Could you check a few things on this drawing? It's one solid part, dimensions in mm from its lowest x, y, z. Coordinates: 2 decimals unless noted, no trailing zeros. Order: outer loops, then holes, each group sorted by start corner. A loop starts at its lowest first (then second) coordinate and runs counter-clockwise, first axis right, second up.
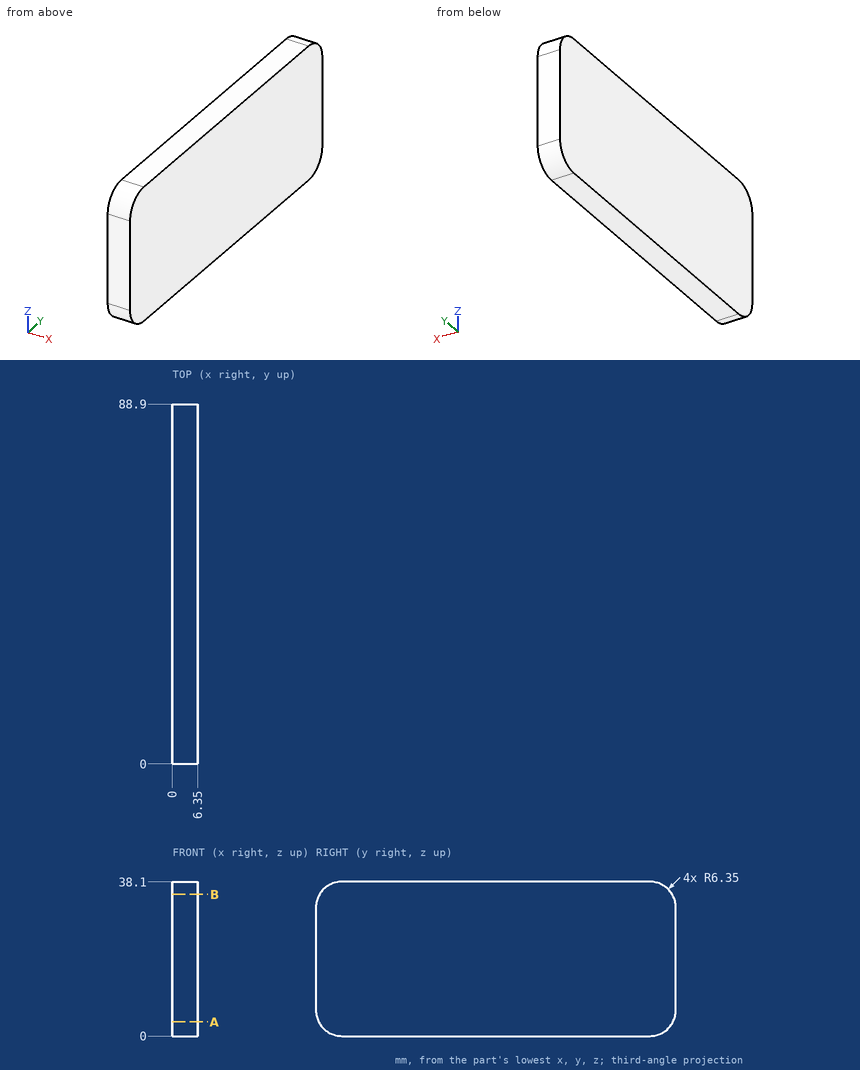
Item 1: Suppose I cut it at A-A (z = 3.5). List the corners of the cut face in (x, y) for me.
Item 2: Suppose I cut it at B-B (z = 35). List the corners of the cut face in (x, y) for me, and give its area (3 significant figures).
Item 3: I need wall thicknesses on line 1 (Y direction, x = 5, z = 2.5); line 2 (Y direction, x = 5.25, z = 3.5). Which ranges of each line are inside material? Lowest first, please.
Geometry results:
1. outline: (0, 0.68) - (6.35, 0.68) - (6.35, 88.22) - (0, 88.22) - close
2. outline: (0, 0.89) - (6.35, 0.89) - (6.35, 88.01) - (0, 88.01) - close
2. area: 553 mm2
3. line 1: y = 1.3 to 87.6
3. line 2: y = 0.68 to 88.22
